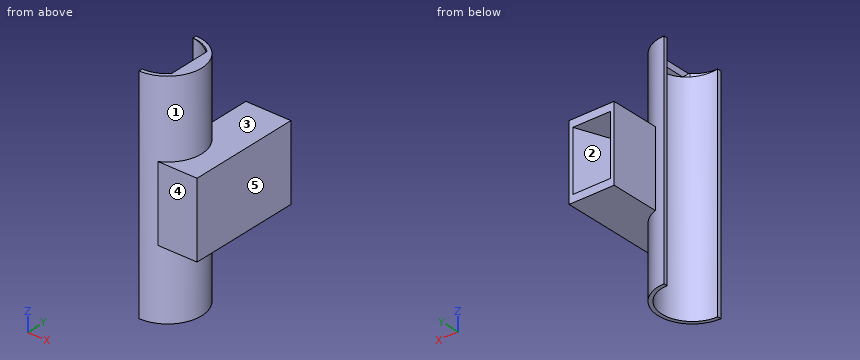
from build123d import *

# Parameters (mm, degrees)
F1_DEPTH     = 37.95141
F3_DEPTH     = 0.75946
F4_T4_DEPTH  = 76.9415838332
F4_S5_R      = 10.287
F4_T6_DEPTH  = 40
F5_W         = 23.114
F5_H         = 1.59512
F6_DEPTH     = 25.4
F9_DEPTH     = 25.4
F10_T4_DEPTH = 21.5531370707
F10_S5_R     = 10.287
F10_T6_DEPTH = 12
F14_W        = 15.24
F14_H        = 25.4
F14_W_2      = 12.7
F14_H_2      = 20.32
F15_DEPTH    = 38.1
F12_W        = 6.096
F12_H        = 20.32
F17_DEPTH    = 25.4


# Not quite as in the source:
# - a fillet or chamfer that OpenCascade refuses, or shapes differently, is made with other operations: its cross-section is extruded or revolved along the edge and cut away or added


with BuildPart() as f1:
    # F0 (on Top) → F1 (new body, symmetric)
    with BuildSketch(Plane.XY):
        with BuildLine():
            ThreePointArc((0, 10.287), (10.287, 0), (0, -10.287))
            Line((0, -10.287), (0, -11.557))
            ThreePointArc((0, -11.557), (11.557, 0), (0, 11.557))
            Line((0, 11.557), (0, 10.287))
        make_face()
    extrude(amount=F1_DEPTH, both=True)

    # F2 (on face) → F3 (join, symmetric)
    with BuildSketch(Plane.XY.offset(37.95141)):
        with BuildLine():
            Line((0, 11.557), (0, -11.557))
            ThreePointArc((0, -11.557), (11.557, 0), (0, 11.557))
        make_face()
    extrude(amount=F3_DEPTH, both=True)

    # F4: chamfer of 1.524 x 10.8438234569 on 1 edges, made by hand


with BuildPart() as f4_tool2:
    # F4_s3 → F4_t4 (new body)
    with BuildSketch(Plane.XZ.offset(-38.4707919166)):
        Polygon((0, 38.71595), (10.8438234569, 37.19195), (0, 37.19195), align=None)
    extrude(amount=F4_T4_DEPTH)

    # F4_s5 → F4_t6 (intersect, symmetric)
    with BuildSketch(Plane.XY.offset(38)):
        Circle(F4_S5_R)
    extrude(amount=F4_T6_DEPTH, both=True, mode=Mode.INTERSECT)


with BuildPart() as f1_1:
    add(f1.part)

    # F4_t1: cut F4_tool2
    add(f4_tool2.part, mode=Mode.SUBTRACT)

    # F5 (on face) → F6 (cut)
    with BuildSketch(Plane(origin=(0, 0, 0), x_dir=(0, -1, 0), z_dir=(-1, 0, 0))):
        with Locations((0, -37.15385)):
            Rectangle(F5_W, F5_H)
    extrude(amount=-F6_DEPTH, mode=Mode.SUBTRACT)

    # F8 (on face) → F9 (cut)
    with BuildSketch(Plane.XY.offset(38.71087)):
        with BuildLine():
            Line((7.0719993682, -7.4705551291), (6.9994361845, 7.5385848871))
            ThreePointArc((6.9994361845, 7.5385848871), (3.7766669941, 9.5686548384), (0.0361460782, 10.2869364954))
            Line((0.0361460782, 10.2869364954), (0.0361460782, -10.2869364954))
            ThreePointArc((0.0361460782, -10.2869364954), (3.8228829333, -9.5502845548), (7.0719993682, -7.4705551291))
        make_face()
    extrude(amount=-F9_DEPTH, mode=Mode.SUBTRACT)

    # F10: chamfer of 1.27 on 1 edges, made by hand


with BuildPart() as f10_tool2:
    # F10_s3 → F10_t4 (new body)
    with BuildSketch(Plane(origin=(0.0519758467, -10.7508066832, -0.0073047289), x_dir=(-0.9999883135, -0.0048345432, 0), z_dir=(-0.0048345421, 0.9999880827, 0.0006794506))):
        with BuildLine():
            Line((-7.0024721698, 39.0354748619), (-8.3267685678, 37.5120486506))
            Line((-8.3267685678, 37.5120486506), (-8.3232336123, 37.4868958359))
            ThreePointArc((-8.3232336123, 37.4868958359), (-7.6800684701, 37.6109410786), (-7.0322650445, 37.7019828278))
            Line((-7.0322650445, 37.7019828278), (-7.0104, 37.7271356426))
            ThreePointArc((-7.0104, 37.7271356426), (-7.0104, 38.3813052522), (-6.9770721698, 39.0354748619))
            Line((-6.9770721698, 39.0354748619), (-7.0024721698, 39.0354748619))
        make_face()
    extrude(amount=F10_T4_DEPTH)

    # F10_s5 → F10_t6 (intersect, symmetric)
    with BuildSketch(Plane.XY.offset(38.3)):
        Circle(F10_S5_R)
    extrude(amount=F10_T6_DEPTH, both=True, mode=Mode.INTERSECT)


with BuildPart() as f1_2:
    add(f1_1.part)

    # F10_t1: cut F10_tool2
    add(f10_tool2.part, mode=Mode.SUBTRACT)

    # F14 (on offset) → F15 (join)
    with BuildSketch(Plane.XZ.offset(-27.8384)):
        with Locations((10.922, 0)):
            Rectangle(F14_W, F14_H)
        with Locations((10.922, 0)):
            Rectangle(F14_W_2, F14_H_2, mode=Mode.SUBTRACT)
        with Locations((10.922, 0)):
            Rectangle(F14_W_2, F14_H_2)
    extrude(amount=F15_DEPTH)

    # F14 (on offset) → F16 section 0
    with BuildSketch(Plane.XZ.offset(-27.8384)):
        with Locations((10.922, 0)):
            Rectangle(F14_W_2, F14_H_2)
    # F12 (on offset) → F16 section 1
    with BuildSketch(Plane.XZ.offset(-10.16)):
        with Locations((7.62, 0)):
            Rectangle(F12_W, F12_H)
    loft(mode=Mode.SUBTRACT)

    # F17 (cut): a face of the model
    f17_faces = [f1_2.faces().sort_by_distance(p)[0] for p in [
        (6.1976073011, 0, -12.7),
    ]]
    extrude(f17_faces, amount=-F17_DEPTH, mode=Mode.SUBTRACT)


solid = f1_2.part
Input: part model. Units: mm. Frame: model coordinates. Face numbers are marked on the shaded views. A direction names the side the tool comes from. Round coordinates to 2 decimals unless told otherwise and drop trailing zeros. Order: outer loops, then holes, each group sorted by start corner. A loop starts at its lowest first (then second) coordinate and runs counter-clockwise, first axis right, second up. Notation, with made-up numbers: (-33.75, 18.25) - (13.25, 18.25) arc R28 cw to (13.25, 43.25) - close; hole circle Ø1 at (18, -15). An arc over 180 degrees is marked (long way). Use a Markdown table: item, result.
1. First-contact query: pin 1 (6 mm diameter, centred on x = 5, y = 14, fed in from -Z); pin 2 (6 mm diameter, centred on y = 21, z = -10, fed in from -X); pin 3 (12 mm diameter, centred on y = 0.5, z = 2, fed in from -X). Flat tips, straight axial feed; report the tip coordinate or a pass-through.
Evaluation:
| item | result |
|---|---|
| pin 1 | z = -12.7 |
| pin 2 | x = 3.3 |
| pin 3 | x = 7.97 |
2. Section A-A on y = 0. Return the cut outline in (x, z).
Evaluation:
| item | result |
|---|---|
| outline | (7.28, 38.71) - (8.29, 37.55) - (10.29, 37.27) - (10.29, -36.36) - (11.56, -36.36) - (11.56, -12.7) - (18.54, -12.7) - (18.54, 12.7) - (11.56, 12.7) - (11.56, 38.71) - close |
3. Section B-B on z = -19. Return the cut outline in (x, y).
Evaluation:
| item | result |
|---|---|
| outline | (0, -11.56) arc R11.56 ccw to (0, 11.56) - (0, 10.29) arc R10.29 cw to (0, -10.29) - close |
4. Access query for the marked faces 4 and 5. Directions: +Z, -Z, +X, -X, +Y, -Y. A direction counts if a zero-diameter tool reaches every point of the face in a straight line with its end or side. Return the directions, or none.
Evaluation:
| item | result |
|---|---|
| face 4 | +Z, -Z, +X, -Y |
| face 5 | +Z, -Z, +X, +Y, -Y |
5. Mould query, pull axis Z, two halves, no side actions, for the marked faces 1, 2 and 3. Classes: +Z half, -Z half, draft (parallel to the pull), parting line (faces both ways), or undercut.
Evaluation:
| item | result |
|---|---|
| face 1 | draft |
| face 2 | undercut |
| face 3 | +Z half |
6. Material intervals for probe 1 along Z at (x, y) = (8.25, 14); probe 2 along Z at (x, y) = (17, 15); probe 3 along Y at (x, z) = (5.5, 6), sorted ascending.
Evaluation:
| item | result |
|---|---|
| probe 1 | -12.7 to -10.16, 10.16 to 12.7 |
| probe 2 | -12.7 to 12.7 |
| probe 3 | -10.26 to -8.69, 8.69 to 10.16 |
